Drawing for the job (mm, zero at the part's lowest x, y, z). Give positions to 0.01 mm unless a question says otherwise; leave off trailing zeros. Order: outer loops, then holes, each group sorted by start corner. A loop starts at its lowest first (then second) coordinate and runs counter-clockwise, first axis right, second up. Notation, with made-up numbers: (-34.75, 60.5) - (-7.75, 60.5) arc R18 cw to (-7.75, 95.5) - close; hole circle Ø6 at (54.25, -3). An arc over 180 degrees is marked (long way). Use a Markdown table: item, result. Add a question column.
(1) Slice it at D-D (z = 5). Write the cut outline in (x, y), then the cut area to 3 significant figures.
(2) Slice it at C-C (x = 38). Write the cut outline in (y, z), then the cut area to 3 significant figures.
(3) Slice it at A-A (x = 8). Write the cut outline in (y, z), then the cut area to 3 significant figures.
(4) Mould opens along Y. For the marked faces 1, 2 and 3 say: +Y half, -Y half, draft (parallel to the pull), parting line (faces both ways), or undercut.
(5) Wall check: line 1 (Y direction, x = 38, z = 7.5); line 2 (Y direction, x = 11, z = 5); line 3 (Y direction, x = 9.25, z = 5). Give the ranges that are in metal, low to high.
(6) Slice it at B-B (y = 39). Write the cut outline in (x, z).
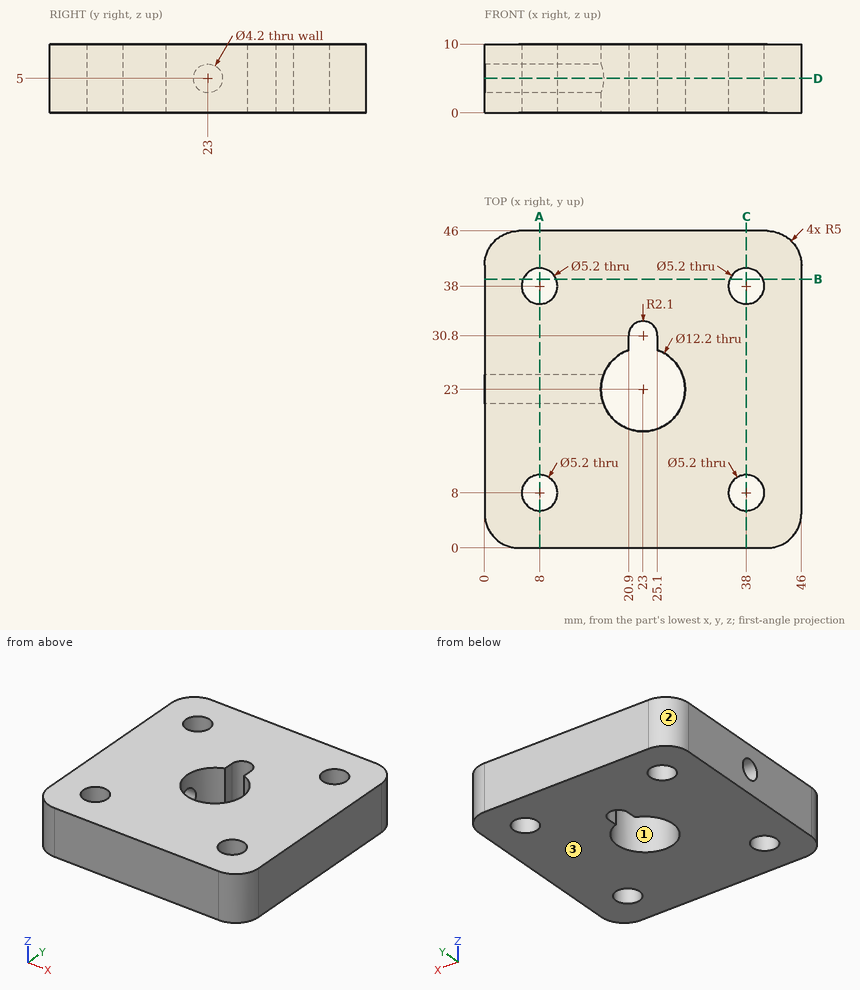
Solution:
| question | item | result |
|---|---|---|
| 1 | outline | (0, 5) arc R5 ccw to (5, 0) - (41, 0) arc R5 ccw to (46, 5) - (46, 41) arc R5 ccw to (41, 46) - (5, 46) arc R5 ccw to (0, 41) - (0, 25.1) - (17.27, 25.1) arc R6.1 cw to (20.9, 28.73) - (20.9, 30.8) arc R2.1 cw to (25.1, 30.8) - (25.1, 28.73) arc R6.1 cw (long way) to (17.27, 20.9) - (0, 20.9) - close; hole circle Ø5.2 at (8, 8); hole circle Ø5.2 at (8, 38); hole circle Ø5.2 at (38, 8); hole circle Ø5.2 at (38, 38) |
| 1 | area | 1,810 mm2 |
| 2 | outline | (0, 0) - (5.4, 0) - (5.4, 10) - (0, 10) - close; (10.6, 0) - (35.4, 0) - (35.4, 10) - (10.6, 10) - close; (40.6, 0) - (46, 0) - (46, 10) - (40.6, 10) - close |
| 2 | area | 356 mm2 |
| 3 | outline | (0, 0) - (5.4, 0) - (5.4, 10) - (0, 10) - close; (10.6, 0) - (35.4, 0) - (35.4, 10) - (10.6, 10) - close; (40.6, 0) - (46, 0) - (46, 10) - (40.6, 10) - close; hole circle Ø4.2 at (23, 5) |
| 3 | area | 342 mm2 |
| 4 | face 1 | undercut |
| 4 | face 2 | +Y half |
| 4 | face 3 | draft |
| 5 | line 1 | 0 to 5.4, 10.6 to 35.4, 40.6 to 46 |
| 5 | line 2 | 0 to 20.9, 25.1 to 46 |
| 5 | line 3 | 0 to 5.72, 10.28 to 20.9, 25.1 to 35.72, 40.28 to 46 |
| 6 | outline | (0, 0) - (5.6, 0) - (5.6, 10) - (0, 10) - close; (10.4, 0) - (35.6, 0) - (35.6, 10) - (10.4, 10) - close; (40.4, 0) - (46, 0) - (46, 10) - (40.4, 10) - close |
